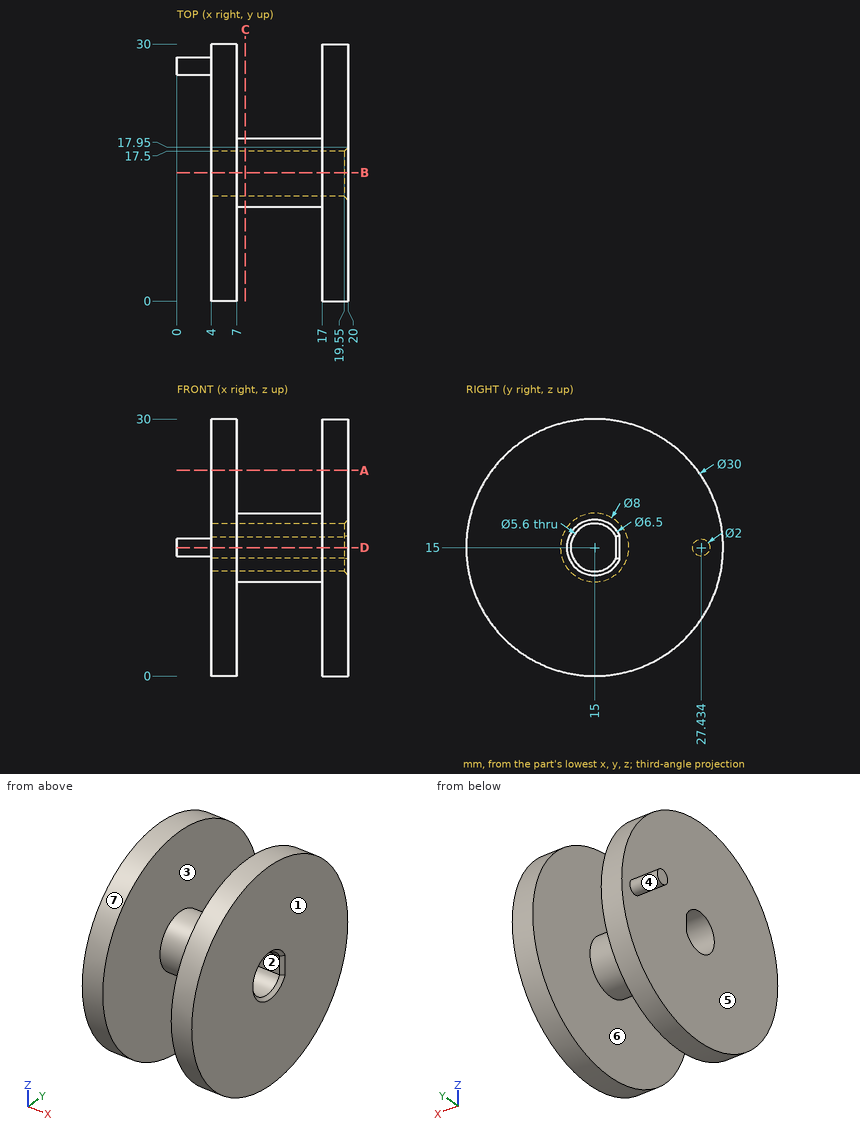
The figure shows three views and two pictorial views of one solid part (mm, origin at its lowest corner). Answer the questions. A direction names the side the tool comes from. Round coordinates to 2 decimals unless told otherwise and drop trailing zeros. Order: outer loops, then holes, each group sorted by start corner. A loop starts at its lowest first (then second) coordinate and runs counter-clockwise, first axis right, second up. Notation, with made-up numbers: M -28.75,66.5 L 18.25,66.5 A24 cw 18.25,83.5 Z; hole C -16.75,-17 d3. An arc over 180 degrees is marked long. Answer in a Markdown table with one row per item. Add a question column.
1) Determine the mould class of the marked faces 5, 6 and 7 for opening direction X: pulls with the +X half, pulls with the -X half, needs draft (parallel to the pull), parting line crosses it, or undercut.
2) Consider line 1 along X through (y, z) = (17, 6.5); line 2 along Y through (x, z) = (11.5, 15); line 3 along Y through (x, z) = (14, 13.25) (1 decimal). Determine where each line is inside the solid, lowest interval first. Write a range as from..to.
3) The part is cut by section A-A on z = 24. Determine the outline of the cut face in (x, y), plus the area to 3 significant figures.
4) The part is cut by section B-B on y = 15. Determine the outline of the cut face in (x, z).
5) The part is cut by section D-D on z = 15. Determine the outline of the cut face in (x, y), plus the area to 3 significant figures.
6) The part is cut by section C-C on x = 8. Determine the outline of the cut face in (y, z).
7) Which of the six approach directions +Z, -Z, +X, -X, +Y, -Y give full straight-line access (tool end or side, diameter ignored) to the marked faces 1, 2, 3 and 4?
8) Flat-ended cylindrical pins translate along their axes: pin 1 Ø3 at (x, z) = (11, 15) entering from -Y; pin 2 Ø1 at (y, z) = (9, 11) entering from -X; pin 3 Ø8 at (x, z) = (9.5, 8.5) entering from +Y (1 decimal). Find the tip coordinate at first contact, or state that the pin passes through.
Findings below:
| question | item | result |
|---|---|---|
| 1 | face 5 | pulls with the -X half |
| 1 | face 6 | undercut |
| 1 | face 7 | needs draft |
| 2 | line 1 | x = 4..7, 17..20 |
| 2 | line 2 | y = 11..12.2, 17.5..19 |
| 2 | line 3 | y = 11.4..12.8, 17.2..18.6 |
| 3 | outline | M 4,3 L 7,3 L 7,27 L 4,27 Z; M 17,3 L 20,3 L 20,27 L 17,27 Z |
| 3 | area | 144 mm² |
| 4 | outline | M 4,0 L 7,0 L 7,11 L 17,11 L 17,0 L 20,0 L 20,11.75 L 19.55,12.2 L 4,12.2 Z; M 4,17.8 L 19.55,17.8 L 20,18.25 L 20,30 L 17,30 L 17,19 L 7,19 L 7,30 L 4,30 Z |
| 5 | outline | M 0,26.43 L 4,26.43 L 4,17.5 L 19.55,17.5 L 20,17.95 L 20,30 L 17,30 L 17,19 L 7,19 L 7,30 L 4,30 L 4,28.43 L 0,28.43 Z; M 4,0 L 7,0 L 7,11 L 17,11 L 17,0 L 20,0 L 20,11.75 L 19.55,12.2 L 4,12.2 Z |
| 5 | area | 183 mm² |
| 6 | outline | C 15,15 d8; hole M 17.5,13.74 L 17.5,16.26 A2.8 ccw long Z |
| 7 | face 1 | +Z, -Z, +X, +Y, -Y |
| 7 | face 2 | +X, -X |
| 7 | face 3 | none |
| 7 | face 4 | -X |
| 8 | pin 1 | stops at y = 11 |
| 8 | pin 2 | stops at x = 4 |
| 8 | pin 3 | stops at y = 29.6 |
